Source: CAD feature listing. Evaluate the final solid. Frame: model axes, mm. A direction names the side the tool comes from. Round coordinates to 2 decimals unless told otherwise and drop trailing zeros. Order: outer loops, then holes, each group sorted by start corner. A loop starts at its lowest first (then second) coordinate and runs counter-clockwise, first axis right, second up.
```python
from build123d import *

# Parameters (mm, degrees)
F1_DEPTH = 5


with BuildPart() as f1:
    # F0 (on Front) → F1 (new body)
    with BuildSketch(Plane.XZ):
        with BuildLine():
            Line((8.335973, -94.735098), (8.335973, 35.264902))
            Line((8.335973, 35.264902), (-27.632447, 35.264902))
            ThreePointArc((-27.632447, 35.264902), (-33.632447, 33.279139), (-37.263132, 28.105998))
            Line((-37.263132, 28.105998), (-36.180024, -87.812574))
            ThreePointArc((-36.180024, -87.812574), (-32.936412, -92.545844), (-27.632447, -94.735098))
            Line((-27.632447, -94.735098), (8.335973, -94.735098))
        make_face()
        Polygon((-17.00996, -26.853288), (-17.00996, -18.853288), (-11.00996, -18.853288), (-11.00996, -26.853288), (-3.239573, -26.853288), (-3.239573, -32.853288), (-11.00996, -32.853288), (-11.00996, -40.853288), (-17.00996, -40.853288), (-17.00996, -32.853288), (-24.780346, -32.853288), (-24.780346, -26.853288), align=None, mode=Mode.SUBTRACT)
    extrude(amount=F1_DEPTH)


solid = f1.part
```
1. Section C-C on z = -21.5. Return loops of the section in (x, y), plus the area to 3 significant figures.
2. Section B-B on x = -6. Return loops of the section in (y, z).
3. Section A-A on y = -3.6. Return loops of the section in (x, z), plus the area to 3 significant figures.
4. Pull-direction query (X, two-part tool) for faces 3 (the face through (-21, -2, -32.853)), 4 (the face through (8.336, -2, -31)), 5 (the face through (-25, -5, -29)); classes: released by +X, released by -X, zero draft, split by the parting line, or undercut.
5. Line query: line 1 along Z through (x, y) = (-19, -1.4); line 2 along Z through (x, y) = (-15, -4.7); line 3 along X through (y, z) = (-0.9, -85). Output: solid intervals per line, ascending.
6. Access query for faces 1 (the face through (-17.01, -2, -37)), 2 (the face through (-25, 0, -29)). Directions: +Z, -Z, +X, -X, +Y, -Y. A direction counts if a zero-diameter tool reaches every point of the face in a straight line with its end or side. Return the directions, or none.
7. First-contact query: pin 1 (2 mm diameter, centred on y = -1.5, z = 13.5, fed in from -X); pin 2 (1.5 mm diameter, centred on y = -2, z = -30, fed in from -X). Flat tips, straight axial feed; report the tip coordinate or a pass-through.
Result:
1. outline: (-36.8, -5) - (-17.01, -5) - (-17.01, 0) - (-36.8, 0) - close; (-11.01, -5) - (8.34, -5) - (8.34, 0) - (-11.01, 0) - close
1. area: 196 mm2
2. outline: (-5, -94.74) - (0, -94.74) - (0, -32.85) - (-5, -32.85) - close; (-5, -26.85) - (0, -26.85) - (0, 35.26) - (-5, 35.26) - close
3. outline: (-37.26, 28.11) - (-36.18, -87.81) arc R10.06 ccw to (-27.63, -94.74) - (8.34, -94.74) - (8.34, 35.26) - (-27.63, 35.26) arc R10.06 ccw to start; hole (-24.78, -32.85) - (-17.01, -32.85) - (-17.01, -40.85) - (-11.01, -40.85) - (-11.01, -32.85) - (-3.24, -32.85) - (-3.24, -26.85) - (-11.01, -26.85) - (-11.01, -18.85) - (-17.01, -18.85) - (-17.01, -26.85) - (-24.78, -26.85) - close
3. area: 5,600 mm2
4. face 3: undercut
4. face 4: released by +X
4. face 5: zero draft
5. line 1: z = -94.74 to -32.85, -26.85 to 35.26
5. line 2: z = -94.74 to -40.85, -18.85 to 35.26
5. line 3: x = -36.21 to 8.34
6. face 1: +Y, -Y
6. face 2: +Z, -Z, +X, -X, +Y
7. pin 1: stops at x = -37.14
7. pin 2: stops at x = -36.73
